```python
from build123d import *

# Parameters (mm, degrees)
SKETCH1_W           = 45
SKETCH1_H           = 12.5
BOSS_EXTRUDE1_DEPTH = 2
SKETCH2_W           = 45
SKETCH2_H           = 37
BOSS_EXTRUDE2_DEPTH = 2
FILLET1_R           = 1
FILLET2_R           = 3


with BuildPart() as part:
    # Sketch1 → Boss-Extrude1 (new body)
    with BuildSketch(Plane(origin=(0, 0, 0), x_dir=(1, 0, 0), z_dir=(0, 1, 0))):
        with Locations((22.5, 6.25)):
            Rectangle(SKETCH1_W, SKETCH1_H)
    extrude(amount=BOSS_EXTRUDE1_DEPTH)

    # Sketch2 → Boss-Extrude2 (add)
    with BuildSketch(Plane(origin=(0, 0, -12.5), x_dir=(-1, 0, 0), z_dir=(0, 0, -1))):
        with Locations((-22.5, 20.5)):
            Rectangle(SKETCH2_W, SKETCH2_H)
    extrude(amount=-BOSS_EXTRUDE2_DEPTH)

    # Fillet1
    fillet1_edges = [part.edges().sort_by_distance(p)[0] for p in [
        (22.5, 2, -10.5),
    ]]
    fillet(fillet1_edges, radius=FILLET1_R)

    # Fillet2
    fillet2_edges = [part.edges().sort_by_distance(p)[0] for p in [
        (22.5, 0, -12.5),
    ]]
    fillet(fillet2_edges, radius=FILLET2_R)


solid = part.part
```
For this review, take the finished solid that the model builds, in its own axes (mm). A direction names the side the tool comes from. Coordinates: 2 decimals unless noted, no trailing zeros. Write each loop counter-clockwise with the first axis right and the second up, starting at its lowest first coordinate (ties: lowest second). Pieces come first, ordered by that corner, then holes.
(1) Wall thickness on probe 1 along Z at (x, y) = (24, 12); probe 2 along Y at (x, z) = (10, -9.25); probe 3 along Z at (x, y) = (32, 2.5): over which ranges is each line inside the solid? List them lowest first.
(2) For pin 1 Ø3 at (x, z) = (18.5, -6) entering from +Y; pin 2 Ø12 at (x, y) = (19.5, 34) entering from +Z, all flat-tipped, find the tip position at first contact; note any pin that passes through.
(3) Add section C-C on z = -0.75. Give the boundary of the cut face in (x, y), then the cut area to 3 significant figures.
(4) Add section B-B on y = 19.5. Give the boundary of the cut face in (x, z), then the cut area to 3 significant figures.
(5) Add section A-A on x = 33. Give the boundary of the cut face in (y, z).
(6) Tool access review of faces 1 (the face through (22, 1, 0)), 2 (the face through (23, 21, -10.5)): name each direction out of +Z, -Z, +X, -X, +Y, -Y from which nothing blocks a thin tool from reaching the whole face with its end or side.
Answer sheet:
1. probe 1: z = -12.5 to -10.5
1. probe 2: y = 0 to 2
1. probe 3: z = -12.46 to -10.37
2. pin 1: stops at y = 2
2. pin 2: stops at z = -10.5
3. outline: (0, 0) - (45, 0) - (45, 2) - (0, 2) - close
3. area: 90.0 mm2
4. outline: (0, -12.5) - (45, -12.5) - (45, -10.5) - (0, -10.5) - close
4. area: 90.0 mm2
5. outline: (0, -9.5) arc R3 ccw to (3, -12.5) - (39, -12.5) - (39, -10.5) - (3, -10.5) arc R1 cw to (2, -9.5) - (2, 0) - (0, 0) - close
6. face 1: +Z, +X, -X, +Y, -Y
6. face 2: +Z, +X, -X, +Y
